For this review, take the finished solid that the model builds, in its own axes (mm). Face numbers are marked on the shaded views. A direction names the side the tool comes from. Coordinates: 2 decimals unless noted, no trailing zeros. Order: outer loops, then holes, each group sorted by start corner. A loop starts at its lowest first (then second) coordinate and runs counter-clockwise, first axis right, second up. Notation, with made-up numbers: (72, 66.5) -> (100, 66.5) arc R12 ccw to (100, 87.5) -> close; hole circle Ø5 at (-2.5, -17.75). An arc over 180 degrees is marked (long way). Write item = value, one per line. Start each with the question number.
1) Machinability: for the marked faces 1 and 2, which of the approach directions +Z, -Z, +X, -X, +Y, -Y give a long, thin tool a straight path to every point of the face, cutting with its end or side? Answer none if there is none.
2) Wall thickness on probe 1 along Y at (x, z) = (18.15, 12.7) (1 decimal); probe 2 along X at (y, z) = (17.5, -57.5) (3 decimals); probe 3 along Y at (x, z) = (3.25, -31) (3 decimals): over which ranges is each line inside the solid? List them lowest first. Write a range as [from, to].
3) Consider section A-A on x = 9.75. Give the boundary of the cut face in (y, z) (3 decimals), and give its area (3 significant figures).
4) Draft analysis for pull direction X (two halves, no side actions). For the marked faces 3, 4 and 5, state which applies: +X half, -X half, draft (parallel to the pull), parting line (faces both ways), or undercut.
5) Insertion check: pin 1 Ø1.2 at (x, y) = (1.5, 18) entering from -Z; pin 2 Ø1.2 at (x, y) = (18, 17.5) entering from -Z; pin 3 Ø5 at (y, z) = (10, 10) entering from +X; pin 4 Ø7.5 at (y, z) = (12.7, 12.7) entering from +X. Each pin has a flat end and moves straight along its axis. Give the tip position at first contact, or say it passes through.
6) Consider section C-C on y = 14.5. Give the boundary of the cut face in (x, z) (3 decimals).
7) Consider section D-D on y = 9.75. Give the boundary of the cut face in (x, z) (3 decimals).
8) Consider section B-B on z = -9.5. Give the boundary of the cut face in (x, y) (3 decimals), and give its area (3 significant figures).
from build123d import *

# Parameters (mm, degrees)
BOSS_EXTRUDE1_DEPTH = 19.05
SKETCH2_W           = 12.7
SKETCH2_H           = 12.7
CUT_EXTRUDE3_DEPTH  = 106.732743864
SKETCH3_W           = 19.05
SKETCH3_H           = 19.05
SKETCH3_W_2         = 12.7
SKETCH3_H_2         = 12.7
BOSS_EXTRUDE2_DEPTH = 12.7
CUT_EXTRUDE5_DEPTH  = 19.05


with BuildPart() as part:
    # Sketch1 → Boss-Extrude1 (new body)
    with BuildSketch(Plane(origin=(0, 0, 0), x_dir=(0, 0, -1), z_dir=(1, 0, 0))):
        Polygon((-12.7, 22.225), (81.966367037, 22.225), (88.9, 22.225), (81.966367037, 3.175), (-12.7, 3.175), align=None)
    extrude(amount=BOSS_EXTRUDE1_DEPTH)

    # Sketch2 → Cut-Extrude3 (cut, through all)
    with BuildSketch(Plane.XY.offset(12.7)):
        with Locations((9.525, 12.7)):
            Rectangle(SKETCH2_W, SKETCH2_H)
    extrude(amount=-CUT_EXTRUDE3_DEPTH, mode=Mode.SUBTRACT)

    # Sketch3 → Boss-Extrude2 (add)
    with BuildSketch(Plane.XY.offset(12.7)):
        with Locations((9.525, 12.7)):
            Rectangle(SKETCH3_W, SKETCH3_H)
        with Locations((9.525, 12.7)):
            Rectangle(SKETCH3_W_2, SKETCH3_H_2, mode=Mode.SUBTRACT)
    extrude(amount=BOSS_EXTRUDE2_DEPTH)

    # Sketch4 → Cut-Extrude5 (cut)
    with BuildSketch(Plane(origin=(19.05, 0, 0), x_dir=(0, 0, -1), z_dir=(1, 0, 0))):
        with BuildLine():
            Line((-11.7, 17.356329697), (-11.7, 16.4625))
            Line((-11.7, 16.4625), (-13.7, 16.4625))
            Line((-13.7, 16.4625), (-13.7, 17.356329697))
            ThreePointArc((-13.7, 17.356329697), (-15.693234559, 8.995684527), (-7.9375, 12.7))
            ThreePointArc((-7.9375, 12.7), (-8.995684527, 15.693234559), (-11.7, 17.356329697))
        make_face()
        with BuildLine():
            Line((-13.7, 16.4625), (-11.7, 16.4625))
            Line((-11.7, 16.4625), (-11.7, 17.356329697))
            ThreePointArc((-11.7, 17.356329697), (-12.7, 17.4625), (-13.7, 17.356329697))
            Line((-13.7, 17.356329697), (-13.7, 16.4625))
        make_face()
        with BuildLine():
            ThreePointArc((-13.7, 17.356329697), (-12.7, 17.4625), (-11.7, 17.356329697))
            Line((-11.7, 17.356329697), (-11.7, 18.4625))
            Line((-11.7, 18.4625), (-13.7, 18.4625))
            Line((-13.7, 18.4625), (-13.7, 17.356329697))
        make_face()
        with BuildLine():
            Line((-25.4, 3.175), (-12.7, 3.175))
            ThreePointArc((-12.7, 3.175), (-22.225, 12.7), (-12.7, 22.225))
            Line((-12.7, 22.225), (-25.4, 22.225))
            Line((-25.4, 22.225), (-25.4, 3.175))
        make_face()
    extrude(amount=-CUT_EXTRUDE5_DEPTH, mode=Mode.SUBTRACT)


solid = part.part
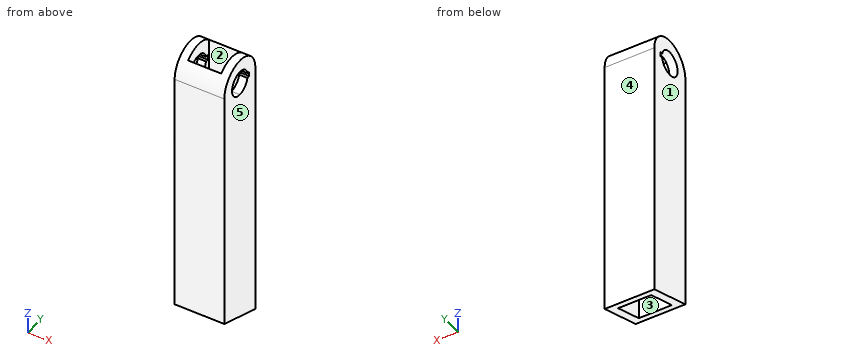
Answer sheet:
q1.face_1 = +Z, -Z, -X, +Y, -Y
q1.face_2 = +Z, -Z
q2.probe_1 = [3.2, 7.9], [18.5, 22.2]
q2.probe_2 = [0, 3.175], [15.875, 19.05]
q2.probe_3 = [3.175, 6.35], [19.05, 22.225]
q3.outline = (3.175, -81.966) -> (6.35, -83.122) -> (6.35, 19.8) arc R9.525 ccw to (3.175, 12.7) -> close; (19.05, -87.744) -> (22.225, -88.9) -> (22.225, 12.7) arc R9.525 ccw to (19.05, 19.8) -> close
q3.area = 654 mm2
q4.face_3 = undercut
q4.face_4 = draft
q4.face_5 = +X half
q5.pin_1 = -87.58
q5.pin_2 = -87.4
q5.pin_3 = 19.05
q5.pin_4 = through
q6.outline = (0, -86.088) -> (3.175, -86.088) -> (3.175, 8.291) -> (0, 8.291) -> close; (0, 17.109) -> (3.175, 17.109) -> (3.175, 22.053) -> (0, 22.053) -> close; (15.875, -86.088) -> (19.05, -86.088) -> (19.05, 8.291) -> (15.875, 8.291) -> close; (15.875, 17.109) -> (19.05, 17.109) -> (19.05, 22.053) -> (15.875, 22.053) -> close
q7.outline = (0, -84.359) -> (3.175, -84.359) -> (3.175, 8.961) -> (0, 8.961) -> close; (0, 16.439) -> (3.175, 16.439) -> (3.175, 21.757) -> (0, 21.757) -> close; (15.875, -84.359) -> (19.05, -84.359) -> (19.05, 8.961) -> (15.875, 8.961) -> close; (15.875, 16.439) -> (19.05, 16.439) -> (19.05, 21.757) -> (15.875, 21.757) -> close
q8.outline = (0, 3.175) -> (19.05, 3.175) -> (19.05, 22.225) -> (0, 22.225) -> close; hole (3.175, 6.35) -> (15.875, 6.35) -> (15.875, 19.05) -> (3.175, 19.05) -> close
q8.area = 202 mm2
